```python
from build123d import *

# Parameters (mm, degrees)
F0_W     = 19.05
F0_H     = 63.5
F1_DEPTH = 1562.1
F3_DEPTH = 63.501
F5_DEPTH = 63.501


with BuildPart() as f1:
    # F0 (on Top) → F1 (new body)
    with BuildSketch(Plane.XY):
        with Locations((9.525, 31.75)):
            Rectangle(F0_W, F0_H)
    extrude(amount=F1_DEPTH)

    # F2 (on face) → F3 (cut, through all)
    with BuildSketch(Plane(origin=(0, 63.5, 0), x_dir=(-1, 0, 0), z_dir=(0, 1, 0))):
        Polygon((0, 19.05), (-19.05, 0), (0, 0), align=None)
    extrude(amount=-F3_DEPTH, mode=Mode.SUBTRACT)

    # F4 (on face) → F5 (cut, through all)
    with BuildSketch(Plane(origin=(0, 63.5, 0), x_dir=(-1, 0, 0), z_dir=(0, 1, 0))):
        Polygon((0, 1562.1), (-19.05, 1562.1), (0, 1543.05), align=None)
    extrude(amount=-F5_DEPTH, mode=Mode.SUBTRACT)


solid = f1.part
```
Source: CAD feature listing. Evaluate the final solid. Frame: model axes, mm. Coordinates: 2 decimals unless noted, no trailing zeros. Loops run counter-clockwise (first coordinate to the right, second up) from the corner with the lowest first, then second, coordinate; pieces in that order, holes last. Notation, with made-up numbers: (39.5, -39.5) -> (88.5, -39.5) arc R29 ccw to (88.5, -2.5) -> close; hole circle Ø2 at (59.5, -35.75). An arc over 180 degrees is marked (long way). One line per item, written item: value. Start each with the question number.
Q1. Line query: line 1 along Z through (x, y) = (2.5, 53); line 2 along Z through (x, y) = (10.5, 55.5). Output: solid intervals per line, ascending.
Q2. Section query A-A, the plane x = 6. Return the cut outline in (y, z), and give its area (3 significant figures).
Q3. Contact query for flat-ended pins moving along their axis: P1, Ø2, axis at x = 9.5, y = 47.5, coming from the +Z side; P2, Ø1, axis at x = 12.5, y = 25.5, coming from the +Z side; P3, Ø6, axis at x = 4, y = 14.5, coming from the +Z side. Output: stop coordinate, or through.
Results:
1. line 1: 16.55 to 1545.55
1. line 2: 8.55 to 1553.55
2. outline: (0, 13.05) -> (63.5, 13.05) -> (63.5, 1549.05) -> (0, 1549.05) -> close
2. area: 97,500 mm^2
3. P1: z = 1553.55
3. P2: z = 1556.05
3. P3: z = 1550.05
